Design review of the part built by this model. Coordinates are the model's own, in mm. Coordinates: 2 decimals unless noted, no trailing zeros. Loops run counter-clockwise (first coordinate to the right, second up) from the corner with the lowest first, then second, coordinate; pieces in that order, holes last.
Q1. Add section B-B on z = 20. Give the boundary of the cut face in (x, y).
Q2. Add section A-A on x = 13.25. Give the boundary of the cut face in (y, z), and give its area (3 significant figures).
Q3. Wall thickness on probe 1 along Z at (x, y) = (3.5, 442); probe 2 along Z at (x, y) = (9.5, 241.5): over which ranges is each line inside the solid? List them lowest first.
Q4. For P1, Ø5, axis at y = 298.5, z = -95, coming from the -X side; P2, Ø4, axis at x = 5, y = -15, coming from the +Z side, all flat-tipped, find the tip position at first contact; note any pin that passes through.
Q5. Add section C-C on y = 275.5. Give the boundary of the cut face in (x, z).
```python
from build123d import *

# Parameters (mm, degrees)
F1_DEPTH = 19.05


with BuildPart() as f1:
    # F0 (on Right) → F1 (new body)
    with BuildSketch(Plane.YZ):
        with BuildLine():
            ThreePointArc((482.6, 127), (467.721024, 162.921024), (431.8, 177.8))
            Line((431.8, 177.8), (-482.6, -152.4))
            ThreePointArc((-482.6, -152.4), (-475.160512, -170.360512), (-457.2, -177.8))
            Line((-457.2, -177.8), (431.8, -177.8))
            ThreePointArc((431.8, -177.8), (467.721024, -162.921024), (482.6, -127))
            Line((482.6, -127), (482.6, 127))
        make_face()
    extrude(amount=F1_DEPTH)


solid = f1.part
```
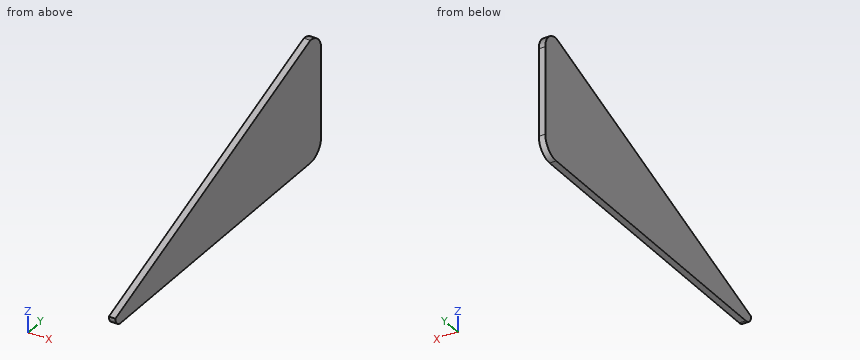
Entries:
1. outline: (0, -5.18) - (19.05, -5.18) - (19.05, 482.6) - (0, 482.6) - close
2. outline: (-482.6, -152.4) arc R25.4 ccw to (-457.2, -177.8) - (431.8, -177.8) arc R50.8 ccw to (482.6, -127) - (482.6, 127) arc R50.8 ccw to (431.8, 177.8) - close
2. area: 191,000 mm2
3. probe 1: z = -176.77 to 176.77
3. probe 2: z = -177.8 to 109.08
4. P1: stops at x = 0
4. P2: stops at z = 17.18
5. outline: (0, -177.8) - (19.05, -177.8) - (19.05, 121.36) - (0, 121.36) - close
